Part model, mm, in its own coordinate system. A direction names the side the tool comes from. Round coordinates to 2 decimals unless told otherwise and drop trailing zeros. Write each loop counter-clockwise with the first axis right and the second up, starting at its lowest first coordinate (ties: lowest second). Pieces come first, ordered by that corner, then holes.
from build123d import *

# Parameters (mm, degrees)
BOSS_EXTRUDE1_DEPTH = 5.3
CIRPATTERN2_COUNT   = 10
SKETCH2_R           = 10
SKETCH2_R_2         = 4
BOSS_EXTRUDE2_DEPTH = 16.6
CUT_EXTRUDE2_START  = -16.6
SKETCH2_2_R         = 4
CUT_EXTRUDE2_DEPTH  = 16.6


with BuildPart() as part:
    # Sketch1 → Boss-Extrude1 (new body)
    with BuildSketch(Plane(origin=(0, 0, 0), x_dir=(0, 0, -1), z_dir=(1, 0, 0))):
        with BuildLine():
            Line((0, 12), (0, 0))
            Line((0, 0), (7.053423028, 9.708203932))
            ThreePointArc((7.053423028, 9.708203932), (5.447885969, 10.692078304), (3.708203874, 11.412678215))
            ThreePointArc((3.708203874, 11.412678215), (1.87721355, 11.852260092), (0, 12))
        make_face()
        with BuildLine():
            ThreePointArc((3.708203874, 11.412678215), (5.447885969, 10.692078304), (7.053423028, 9.708203932))
            Line((7.053423028, 9.708203932), (10.139295602, 13.955543153))
            Line((10.139295602, 13.955543153), (9.935981835, 14.101019997))
            Line((9.935981835, 14.101019997), (6.992185789, 12.620548152))
            ThreePointArc((6.992185789, 12.620548152), (5.559289779, 11.448121491), (3.708203874, 11.412678215))
        make_face()
        with BuildLine():
            Line((0, 17.25), (0, 12))
            ThreePointArc((0, 12), (1.87721355, 11.852260092), (3.708203874, 11.412678215))
            ThreePointArc((3.708203874, 11.412678215), (2.231477037, 12.529393436), (1.761374949, 14.320141621))
            Line((1.761374949, 14.320141621), (0.249993436, 17.248188406))
            ThreePointArc((0.249993436, 17.248188406), (0.125, 17.249547096), (0, 17.25))
        make_face()
    boss_extrude1 = extrude(amount=BOSS_EXTRUDE1_DEPTH)

    # CirPattern2: Boss-Extrude1 ×10 about axis
    cirpattern2_axis = Axis((0, 0, 0), (1, 0, 0))
    for i in range(1, CIRPATTERN2_COUNT):
        add(boss_extrude1.rotate(cirpattern2_axis, i * 360 / CIRPATTERN2_COUNT))

    # Sketch2 → Boss-Extrude2 (add)
    with BuildSketch(Plane.ZY):
        with Locations(Location((0, 0, 0), (0, 0, 180))):
            Circle(SKETCH2_R)
        with Locations(Location((0, 0, 0), (0, 0, 180))):
            Circle(SKETCH2_R_2, mode=Mode.SUBTRACT)
    extrude(amount=BOSS_EXTRUDE2_DEPTH)

    # Sketch2_2 → Cut-Extrude2 (cut)
    with BuildSketch(Plane.ZY.offset(CUT_EXTRUDE2_START)):
        with Locations(Location((0, 0, 0), (0, 0, 180))):
            Circle(SKETCH2_2_R)
    extrude(amount=CUT_EXTRUDE2_DEPTH, mode=Mode.SUBTRACT)


solid = part.part
Q1. Saw through at B-B, the plane y = 9. Write the cut outline in (x, z).
Q2. Drop flat-ended pins along their axis: P1, Ø12, axis at x = -12.5, z = -1, coming from the -Y side; P2, Ø1, axis at x = -7, z = -6.5, coming from the -Y side; P3, Ø4, axis at y = -14, z = -3.5, coming from the -X side. Give the stop position or say it passes through.
Q3. Two-plate mould, pull along Y, no slides. Class faces 5 (the flat face through (2.613, 12.201, 10.095)), 6 (the flat face through (2.61, -5.83, 14.72)), 7 (the flat face through (2.61, 13.35, 8.44)): released by +Y, released by -Y, zero draft, split by the parting line, or undercut.
Q4. Saw through at D-D, the plane y = -0.5. Write the cut outline in (x, z).
Q5. Wall check: line 1 (Y direction, x = -1.25, z = 0); line 2 (Z direction, x = 0.5, y = 12); line 3 (X direction, y = -5, z = 9). Give the ranges that are in metal, low to high.
Q6. Saw through at C-C, the plane x = -9. Write the cut outline in (y, z), and give its area (3 significant figures).
Q7. Tool access for faces 1 (the flat face through (0, -4.3, 9.2)), 2 (the flat face through (2.61, -12.16, 10.09)), 3 (the flat face through (2.61, -13.37, 8.48)), 4 (the flat face through (2.613, -12.201, -10.095)): list every direction of +Z, -Z, +X, -X, +Y, -Y with a clear straight run to the whole face (end or side of a thin tool).
Q8. Saw through at A-A, the plane z = 13.5. Write the cut outline in (x, y), and give its area (3 significant figures).
Computed:
1. outline: (-16.6, -4.36) - (0, -4.36) - (0, -9.18) - (5.3, -9.18) - (5.3, 9.18) - (0, 9.18) - (0, 4.36) - (-16.6, 4.36) - close
2. P1: stops at y = -10
2. P2: stops at y = -8
2. P3: stops at x = 0
3. face 5: undercut
3. face 6: released by -Y
3. face 7: released by +Y
4. outline: (-16.6, -9.99) - (0, -9.99) - (0, -12.04) - (5.3, -12.04) - (5.3, -3.97) - (-16.6, -3.97) - close; (-16.6, 3.97) - (5.3, 3.97) - (5.3, 12.04) - (0, 12.04) - (0, 9.99) - (-16.6, 9.99) - close
5. line 1: y = -10 to -4, 4 to 10
5. line 2: z = -10.06 to -6.47, -2.69 to 2.69, 6.47 to 10.06
5. line 3: x = 0 to 5.3
6. outline: circle Ø20 at (0, 0); hole circle Ø8 at (0, 0)
6. area: 264 mm2
7. face 1: -X
7. face 2: +Z, +X, -X
7. face 3: +X, -X, -Y
7. face 4: -Z, +X, -X
8. outline: (0, -6.03) - (5.3, -6.03) - (5.3, -2.5) - (0, -2.5) - close; (0, 2.5) - (5.3, 2.5) - (5.3, 6.03) - (0, 6.03) - close
8. area: 37.5 mm2
